Read the model definition and answer for the solid it produces. Units are mm, in the model's axes. Coordinates: 2 decimals unless noted, no trailing zeros. Loops run counter-clockwise (first coordinate to the right, second up) from the corner with the lowest first, then second, coordinate; pieces in that order, holes last. Notation, with made-up numbers: (-24.75, -4.75) -> (-17.75, -4.75) arc R25 cw to (-17.75, 17.25) -> close; hole circle Ø8 at (8, -32.75). An arc over 180 degrees is marked (long way). Answer as a JSON object with one key per item and string values. Group by question number.
Q1. The part is cut by section B-B on y = 43. Write down the section's boundary in (x, z), and give its area (3 significant figures).
Q2. The part is cut by section A-A on x = 86. Write down the section's boundary in (y, z), and give its area (3 significant figures).
Q3. Straight lines are drawn through the part: line 1 along Y through (x, z) = (86, 4.5); line 2 along X through (y, z) = (95, 5.5); line 3 along X through (y, z) = (16, 9). For each, find the intervals that lie inside material, in ascending order. Write a range as [from, to].
Q4. The part is cut by section D-D on x = 17. Write down the section's boundary in (y, z), and give its area (3 significant figures).
Q5. Each of these flat-tipped pins is pushed along its axis until it touches: P1, Ø1, axis at x = 22, y = 27.5, coming from the -Z side; P2, Ø8, axis at x = 86, y = 95, coming from the +Z side. Where does it stop, or does it pass through?
Q6. The part is cut by section C-C on z = 10. Write down the section's boundary in (x, y).
Q7. Determine the mould class of faces 1 (the flat face through (49, 110, 6)), 2 (the cylindrical face through (81.504, 15.198, 6.439)), 3 (the flat face through (0, 54, 6)), 4 (the cylindrical face through (14.59, 90.54, 6.44)) for opening direction Y: released by +Y, released by -Y, zero draft, split by the parting line, or undercut.
from build123d import *

# Parameters (mm, degrees)
SKETCH1_W           = 100
SKETCH1_H           = 110
BOSS_EXTRUDE1_DEPTH = 12.7
SKETCH2_R           = 4.5
CUT_EXTRUDE1_DEPTH  = 12.7


with BuildPart() as part:
    # Sketch1 → Boss-Extrude1 (new body)
    with BuildSketch(Plane.XY):
        with Locations((50, 55)):
            Rectangle(SKETCH1_W, SKETCH1_H)
    extrude(amount=BOSS_EXTRUDE1_DEPTH)

    # Sketch2 → Cut-Extrude1 (cut)
    with BuildSketch(Plane.XY.offset(12.7)):
        with Locations((86, 15)):
            Circle(SKETCH2_R)
        with Locations((14, 15)):
            Circle(SKETCH2_R)
        with BuildLine():
            ThreePointArc((18.5, 43), (14, 47.5), (9.5, 43))
            ThreePointArc((9.5, 43), (14, 38.5), (18.5, 43))
        make_face()
        with BuildLine():
            ThreePointArc((18.5, 95), (14, 99.5), (9.5, 95))
            ThreePointArc((9.5, 95), (14, 90.5), (18.5, 95))
        make_face()
        with BuildLine():
            ThreePointArc((90.5, 43), (86, 47.5), (81.5, 43))
            ThreePointArc((81.5, 43), (86, 38.5), (90.5, 43))
        make_face()
        with BuildLine():
            ThreePointArc((90.5, 95), (86, 99.5), (81.5, 95))
            ThreePointArc((81.5, 95), (86, 90.5), (90.5, 95))
        make_face()
    extrude(amount=-CUT_EXTRUDE1_DEPTH, mode=Mode.SUBTRACT)


solid = part.part
Final values:
{
 "1": {"outline": "(0, 0) -> (9.5, 0) -> (9.5, 12.7) -> (0, 12.7) -> close; (18.5, 0) -> (81.5, 0) -> (81.5, 12.7) -> (18.5, 12.7) -> close; (90.5, 0) -> (100, 0) -> (100, 12.7) -> (90.5, 12.7) -> close", "area": "1,040 mm2"},
 "2": {"outline": "(0, 0) -> (10.5, 0) -> (10.5, 12.7) -> (0, 12.7) -> close; (19.5, 0) -> (38.5, 0) -> (38.5, 12.7) -> (19.5, 12.7) -> close; (47.5, 0) -> (90.5, 0) -> (90.5, 12.7) -> (47.5, 12.7) -> close; (99.5, 0) -> (110, 0) -> (110, 12.7) -> (99.5, 12.7) -> close", "area": "1,050 mm2"},
 "3": {"line 1": "y = [0, 10.5], [19.5, 38.5], [47.5, 90.5], [99.5, 110]", "line 2": "x = [0, 9.5], [18.5, 81.5], [90.5, 100]", "line 3": "x = [0, 9.61], [18.39, 81.61], [90.39, 100]"},
 "4": {"outline": "(0, 0) -> (11.65, 0) -> (11.65, 12.7) -> (0, 12.7) -> close; (18.35, 0) -> (39.65, 0) -> (39.65, 12.7) -> (18.35, 12.7) -> close; (46.35, 0) -> (91.65, 0) -> (91.65, 12.7) -> (46.35, 12.7) -> close; (98.35, 0) -> (110, 0) -> (110, 12.7) -> (98.35, 12.7) -> close", "area": "1,140 mm2"},
 "5": {"P1": "stops at z = 0", "P2": "passes through"},
 "6": {"outline": "(0, 0) -> (100, 0) -> (100, 110) -> (0, 110) -> close; hole circle Ø9 at (14, 15); hole circle Ø9 at (14, 43); hole circle Ø9 at (14, 95); hole circle Ø9 at (86, 15); hole circle Ø9 at (86, 43); hole circle Ø9 at (86, 95)"},
 "7": {"face 1": "released by +Y", "face 2": "undercut", "face 3": "zero draft", "face 4": "undercut"}
}
